Verification items for the finished model (mm, model axes). A direction names the side the tool comes from. Round coordinates to 2 decimals unless told otherwise and drop trailing zeros. Order: outer loops, then holes, each group sorted by start corner. A loop starts at its lowest first (then second) coordinate and runs counter-clockwise, first axis right, second up.
```python
from build123d import *

# Parameters (mm, degrees)
SKETCH1_R           = 2.4892
BOSS_EXTRUDE1_DEPTH = 2.794
CUT_EXTRUDE1_DEPTH  = 76.982993088
BOSS_EXTRUDE2_START = -2.794
BOSS_EXTRUDE2_DEPTH = 2.794
CUT_EXTRUDE2_DEPTH  = 93.595404272
FILLET1_R           = 1.5875
FILLET2_R           = 1.5875


with BuildPart() as part:
    # Sketch1 → Boss-Extrude1 (new body)
    with BuildSketch(Plane(origin=(0, 0, 0), x_dir=(0, 0, -1), z_dir=(1, 0, 0))):
        with BuildLine():
            Line((-15.352682977, -58.807991027), (4.499625018, -1.560378463))
            ThreePointArc((4.499625018, -1.560378463), (2.590924963, 3.996062323), (-3.260713933, 3.471188686))
            Line((-3.260713933, 3.471188686), (-40.268643062, -31.292772903))
            ThreePointArc((-40.268643062, -31.292772903), (-42.237439845, -35.268799833), (-41.122639966, -39.563234855))
            Line((-41.122639966, -39.563234855), (-26.553798482, -60.36969678))
            ThreePointArc((-26.553798482, -60.36969678), (-20.475321466, -63.016652797), (-15.352682977, -58.807991027))
        make_face()
        Circle(SKETCH1_R, mode=Mode.SUBTRACT)
        with Locations((-35.921024484, -35.921024484)):
            Circle(SKETCH1_R, mode=Mode.SUBTRACT)
        with Locations((-21.352183001, -56.727486409)):
            Circle(SKETCH1_R, mode=Mode.SUBTRACT)
    extrude(amount=BOSS_EXTRUDE1_DEPTH)

    # Sketch2 → Cut-Extrude1 (cut, through all)
    with BuildSketch(Plane(origin=(2.794, 0, 0), x_dir=(0, 0, -1), z_dir=(1, 0, 0))):
        Polygon((-3.612253937, -5.571289043), (-31.24485752, -31.528395862), (-18.784617945, -49.323462173), align=None)
    extrude(amount=-CUT_EXTRUDE1_DEPTH, mode=Mode.SUBTRACT)

    # Sketch3 → Boss-Extrude2 (add)
    with BuildSketch(Plane(origin=(2.794, 0, 0), x_dir=(0, 0, -1), z_dir=(1, 0, 0)).offset(BOSS_EXTRUDE2_START)):
        with BuildLine():
            Line((-1.562121869, 4.499020062), (-63.85396467, -17.129567629))
            Line((-63.85396467, -17.129567629), (-67.729854308, -31.424790078))
            Line((-67.729854308, -31.424790078), (-57.287773334, -41.92902019))
            Line((-57.287773334, -41.92902019), (-24.697034781, -62.125121685))
            ThreePointArc((-24.697034781, -62.125121685), (-25.714625529, -61.341768064), (-26.553798482, -60.36969678))
            Line((-26.553798482, -60.36969678), (-41.122639966, -39.563234855))
            ThreePointArc((-41.122639966, -39.563234855), (-42.237439845, -35.268799833), (-40.268643062, -31.292772903))
            Line((-40.268643062, -31.292772903), (-3.260713933, 3.471188686))
            ThreePointArc((-3.260713933, 3.471188686), (-2.465572069, 4.074599443), (-1.562121869, 4.499020062))
        make_face()
        Polygon((-56.32839471, -38.390598792), (-45.55447623, -35.537970896), (-42.637965216, -24.781169846), (-50.495372681, -16.876996692), (-61.269291162, -19.729624588), (-64.185802176, -30.486425638), align=None, mode=Mode.SUBTRACT)
    extrude(amount=BOSS_EXTRUDE2_DEPTH)

    # Sketch4 → Cut-Extrude2 (cut, through all)
    with BuildSketch(Plane(origin=(2.794, 0, 0), x_dir=(0, 0, -1), z_dir=(1, 0, 0))):
        Polygon((-41.946495802, -16.24487248), (-34.004795616, -27.58679577), (-10.194346511, -5.220087943), align=None)
    extrude(amount=-CUT_EXTRUDE2_DEPTH, mode=Mode.SUBTRACT)

    # Fillet1
    fillet1_edges = [part.edges().sort_by_distance(p)[0] for p in [
        (1.397, -5.571289043, 3.612253937),
        (1.397, -49.323462173, 18.784617945),
        (1.397, -31.528395862, 31.24485752),
    ]]
    fillet(fillet1_edges, radius=FILLET1_R)

    # Fillet2
    fillet2_edges = [part.edges().sort_by_distance(p)[0] for p in [
        (1.397, -17.129567629, 63.85396467),
        (1.397, -31.424790078, 67.729854308),
        (1.397, -41.92902019, 57.287773334),
        (1.397, -16.24487248, 41.946495802),
        (1.397, -5.220087943, 10.194346511),
        (1.397, -27.58679577, 34.004795616),
    ]]
    fillet(fillet2_edges, radius=FILLET2_R)


solid = part.part
```
1) Sectioned sample at C-C on x = 1. Count the separate pieces of the cut face and the enclosed holes in it, then the cut area to 3 significant figures.
2) Sectioned sample at D-D on z = 37.5. Record the cut outline in (x, y).
3) Scan lines: probe 1 along Z at (x, y) = (0.15, -22); probe 2 along Z at (x, y) = (0.15, -32); probe 3 along Y at (x, z) = (1.15, 27.5). Record each from-to range of solid material in increasing order.
4) Go/stop test with flat-tipped pins: pin 1 Ø1.5 at (x, y) = (1, -42) entering from +Z; pin 2 Ø1 at (x, y) = (1.5, -56) entering from -Z. Record where each tip stops, or that it passes through.
5) Tool access check on faces 1 (the flat face through (1.377, -51.935, 41.14)), 2 (the cylindrical face through (1.377, -31.565, 30.733)). Record the directions out of +Z, -Z, +X, -X, +Y, -Y that give a thin tool (end or side, any length) a straight path to the whole face; none if there is none.
6) Sectioned sample at B-B on z = 0. Record the cut outline in (x, y).
7) Sectioned sample at A-A on y = 0. Record the cut outline in (x, z).
8) Draft check along Y on faces 3 (the cylindrical face through (1.417, -31.351, 67.495)), 4 (the cylindrical face through (1.38, -54.26, 21.68)), 5 (the flat face through (1.377, -36.868, 62.319)). Enter one of: released by +Y, released by -Y, zero draft, split by the parting line, or undercut.
Returned:
1. separate pieces: 1
1. enclosed holes: 6
1. area: 1,800 mm2
2. outline: (0, -54.19) - (2.79, -54.19) - (2.79, -37.85) - (0, -37.85) - close; (0, -34) - (2.79, -34) - (2.79, -22.6) - (0, -22.6) - close; (0, -14.7) - (2.79, -14.7) - (2.79, -7.98) - (0, -7.98) - close
3. probe 1: z = 2.59 to 9.31, 21.1 to 28.06, 37.92 to 45.4, 61.88 to 65.17
3. probe 2: z = 6.06 to 12.78, 30.72 to 44.6, 62.68 to 67.15
3. probe 3: y = -60.39 to -36.88, -28.01 to -21.48, -11.23 to -4.51
4. pin 1: stops at z = 57.96
4. pin 2: stops at z = 14.21
5. face 1: +Z, +X, -X, -Y
5. face 2: +X, -X
6. outline: (0, -14.54) - (2.79, -14.54) - (2.79, -2.49) - (0, -2.49) - close; (0, 2.49) - (2.79, 2.49) - (2.79, 4.76) - (0, 4.76) - close
7. outline: (0, -4.76) - (2.79, -4.76) - (2.79, -2.49) - (0, -2.49) - close; (0, 2.49) - (2.79, 2.49) - (2.79, 14.52) - (0, 14.52) - close
8. face 3: split by the parting line
8. face 4: undercut
8. face 5: released by -Y
